Input: part model. Units: mm. Frame: model coordinates. A direction names the side the tool comes from. Round coordinates to 2 decimals unless told otherwise and drop trailing zeros. Write each loop counter-clockwise with the first axis right and the second up, starting at its lowest first coordinate (ties: lowest second). Pieces come first, ordered by that corner, then holes. Notation, with made-up numbers: M 88.5,-20 L 105.5,-20 A21 ccw 105.5,-10 Z; hole C 5,43 d3. An arc over 180 degrees is marked long. Answer as CSV lines item,"result". Start each with the question number.
```python
from build123d import *

# Parameters (mm, degrees)
F0_W     = 16
F0_H     = 16
F1_DEPTH = 20
F2_W     = 10
F2_H     = 10
F3_DEPTH = 15
F4_R     = 1


with BuildPart() as f1:
    # F0 (on Top) → F1 (new body)
    with BuildSketch(Plane.XY):
        with Locations((-53.225686, -1.982133)):
            Rectangle(F0_W, F0_H)
    extrude(amount=F1_DEPTH)

    # F2 (on face) → F3 (cut)
    with BuildSketch(Plane.XY.offset(20)):
        with Locations((-53.225686, -1.982133)):
            Rectangle(F2_W, F2_H)
    extrude(amount=-F3_DEPTH, mode=Mode.SUBTRACT)

    # F4
    f4_edges = [f1.edges().sort_by_distance(p)[0] for p in [
        (-45.225686, -9.982133, 10),
        (-45.225686, 6.017867, 10),
        (-45.225686, -1.982133, 0),
        (-45.225686, -1.982133, 20),
        (-61.225686, -9.982133, 10),
        (-53.225686, -9.982133, 0),
        (-53.225686, -9.982133, 20),
        (-61.225686, 6.017867, 10),
        (-61.225686, -1.982133, 0),
        (-61.225686, -1.982133, 20),
        (-53.225686, 6.017867, 0),
        (-53.225686, 6.017867, 20),
    ]]
    fillet(f4_edges, radius=F4_R)


solid = f1.part
```
Item 1: Line query: line 1 (X direction, y = -2, z = 13.25); line 2 (Y direction, x = -57.5, z = 5.75); line 3 (Z direction, x = -49, y = 1.5). Output: solid intervals per line, ascending. Write a range as [from, to].
Item 2: Cut plane C-C, the plane y = -3.5. Return loops of the section in (x, z).
Item 3: Pin query (flat end, axial travel): pin 1 Ø5 at (x, y) = (-54, -3.5) entering from +Z. Return the tip coordinate at first contact, or that it passes through.
Item 4: Access query for faces 1 (the face through (-48.226, -2, 13)), 2 (the face through (-60.94, -1.88, 19.7)). Directions: +Z, -Z, +X, -X, +Y, -Y. A direction counts if a zero-diameter tool reaches every point of the face in a straight line with its end or side. Return the directions, or none.
Item 5: Cut plane A-A, the plane z = 13.5. Return loops of the section in (x, y), plus the area to 3 significant figures.
Item 6: Draft query along X for faces 3 (the face through (-53, -2, 5)), 4 (the face through (-60.94, 5.72, 10.13)), 5 (the face through (-53, -9.982, 10)). Return one class per face: +X half, -X half, draft (parallel to the pull), parting line (faces both ways), or undercut.
Item 7: Cut plane B-B, the plane x = -57. Return loops of the section in (y, z), plus the area to 3 significant figures.
Results list:
1,line 1,"[-61.23, -58.23], [-48.23, -45.23]"
1,line 2,"[-9.98, -6.98], [3.02, 6.02]"
1,line 3,"[0, 5]"
2,outline,"M -61.23,1 A1 ccw -60.23,0 L -46.23,0 A1 ccw -45.23,1 L -45.23,19 A1 ccw -46.23,20 L -48.23,20 L -48.23,5 L -58.23,5 L -58.23,20 L -60.23,20 A1 ccw -61.23,19 Z"
3,pin 1,"z = 5"
4,face 1,"+Z"
4,face 2,"+Z, -X, +Y, -Y"
5,outline,"M -61.23,-8.98 A1 ccw -60.23,-9.98 L -46.23,-9.98 A1 ccw -45.23,-8.98 L -45.23,5.02 A1 ccw -46.23,6.02 L -60.23,6.02 A1 ccw -61.23,5.02 Z; hole M -58.23,-6.98 L -48.23,-6.98 L -48.23,3.02 L -58.23,3.02 Z"
5,area,"155 mm²"
6,face 3,"undercut"
6,face 4,"-X half"
6,face 5,"draft"
7,outline,"M -9.98,1 A1 ccw -8.98,0 L 5.02,0 A1 ccw 6.02,1 L 6.02,19 A1 ccw 5.02,20 L 3.02,20 L 3.02,5 L -6.98,5 L -6.98,20 L -8.98,20 A1 ccw -9.98,19 Z"
7,area,"169 mm²"
